Verification items for the finished model (mm, model axes). A direction names the side the tool comes from. Coordinates: 2 decimals unless noted, no trailing zeros. Order: outer loops, then holes, each group sorted by start corner. A loop starts at its lowest first (then second) coordinate and runs counter-clockwise, first axis right, second up.
Q1. Draft check along Y on faces 1 (the cylindrical face through (-0.59, 4.46, 2.65)), 2 (the flat face through (-3, -3, 3.21)), 3 (the flat face through (0, 2, 7)). Enter one of: pulls with the +Y half, pulls with the -Y half, needs draft (parallel to the pull), parting line crosses it, or undercut.
Q2. Cross-section at A-A, the plane y = 0. Record the boundary of the cut face in (x, z).
Q3. Depth check by flat-ended pin: P1, Ø10, axis at x = -0.5, y = 8.5, coming from the +Z side; P2, Ø2, axis at x = -1, z = 6.5, coming from the -Y side; P3, Ø6, axis at y = 4, z = 8.5, coming from the -X side. Enter the tip coordinate at first touch or a pass-through.
Q4. Cross-section at B-B, the plane x = 0. Record the boundary of the cut face in (y, z), and give its area (3 significant figures).
Q5. Cross-section at C-C, the plane z = 9. Record the boundary of the cut face in (x, y).
Q6. Set-up check for faces 4 (the flat face through (2.3, 0, 10.21)), 5 (the flat face through (-1.5, 0, 8)), 6 (the flat face through (-1, 0, 4.21)): record each of +Z, -Z, +X, -X, +Y, -Y from which the full face is reachable in a straight line by a thin tool's end or side.
Q7. Cross-section at D-D, the plane z = 2.75. Record the boundary of the cut face in (x, y), and give its area (3 significant figures).
Q8. Thickness scan on line 1 (Z direction, x = -6.25, y = -4.75); line 2 (Y direction, x = -1, z = 7.25); line 3 (X direction, y = 0.5, z = 8.25). Record the ranges inside material, lowest first.
from build123d import *

# Parameters (mm, degrees)
F0_R     = 11.05
F1_DEPTH = 2.1
F2_R     = 4.5
F3_DEPTH = 1.11
F4_R     = 3.99
F5_DEPTH = 7
F6_W     = 3
F6_H     = 4
F7_DEPTH = 6
F8_W     = 4
F8_H     = 1.5
F9_DEPTH = 1.3
F10_SIZE = 0.5


with BuildPart() as f1:
    # F0 (on Top) → F1 (new body)
    with BuildSketch(Plane.XY):
        Circle(F0_R)
    extrude(amount=F1_DEPTH)

    # F2 (on face) → F3 (join)
    with BuildSketch(Plane.XY.offset(2.1)):
        Circle(F2_R)
    extrude(amount=F3_DEPTH)

    # F4 (on face) → F5 (join)
    with BuildSketch(Plane.XY.offset(3.21)):
        Circle(F4_R)
    extrude(amount=F5_DEPTH)

    # F6 (on face) → F7 (cut)
    with BuildSketch(Plane.XY.offset(10.21)):
        Rectangle(F6_W, F6_H)
    extrude(amount=-F7_DEPTH, mode=Mode.SUBTRACT)

    # F8 (on face) → F9 (cut)
    with BuildSketch(Plane.YZ.offset(-1.5)):
        with Locations((0, 4.96)):
            Rectangle(F8_W, F8_H)
    extrude(amount=-F9_DEPTH, mode=Mode.SUBTRACT)

    # F10
    f10_edges = [f1.edges().sort_by_distance(p)[0] for p in [
        (-1.5, 0, 5.71),
        (0, 2, 10.21),
        (-1.5, 0, 10.21),
        (1.5, 0, 10.21),
        (0, -2, 10.21),
        (-3.99, 0, 10.21),
        (-11.05, 0, 0),
        (-11.05, 0, 2.1),
    ]]
    chamfer(f10_edges, length=F10_SIZE)


solid = f1.part
Check values:
1. face 1: parting line crosses it
1. face 2: needs draft
1. face 3: undercut
2. outline: (-11.05, 0.5) - (-10.55, 0) - (10.55, 0) - (11.05, 0.5) - (11.05, 1.6) - (10.55, 2.1) - (4.5, 2.1) - (4.5, 3.21) - (3.99, 3.21) - (3.99, 9.71) - (3.49, 10.21) - (2, 10.21) - (1.5, 9.71) - (1.5, 4.21) - (-2.8, 4.21) - (-2.8, 5.71) - (-2, 5.71) - (-1.5, 6.21) - (-1.5, 9.71) - (-2, 10.21) - (-3.49, 10.21) - (-3.99, 9.71) - (-3.99, 3.21) - (-4.5, 3.21) - (-4.5, 2.1) - (-10.55, 2.1) - (-11.05, 1.6) - close
3. P1: stops at z = 10.19
3. P2: stops at y = -3.99
3. P3: stops at x = -3.86
4. outline: (-11.05, 0.5) - (-10.55, 0) - (10.55, 0) - (11.05, 0.5) - (11.05, 1.6) - (10.55, 2.1) - (4.5, 2.1) - (4.5, 3.21) - (3.99, 3.21) - (3.99, 9.71) - (3.49, 10.21) - (2.5, 10.21) - (2, 9.71) - (2, 4.21) - (-2, 4.21) - (-2, 9.71) - (-2.5, 10.21) - (-3.49, 10.21) - (-3.99, 9.71) - (-3.99, 3.21) - (-4.5, 3.21) - (-4.5, 2.1) - (-10.55, 2.1) - (-11.05, 1.6) - close
4. area: 87.3 mm2
5. outline: circle Ø7.98 at (0, 0); hole (-1.5, -2) - (1.5, -2) - (1.5, 2) - (-1.5, 2) - close
6. face 4: +Z, +X, -X, +Y, -Y
6. face 5: +Z
6. face 6: none
7. outline: circle Ø9 at (0, 0)
7. area: 63.6 mm2
8. line 1: z = 0 to 2.1
8. line 2: y = -3.86 to -2, 2 to 3.86
8. line 3: x = -3.96 to -1.5, 1.5 to 3.96
